Could you check a few things on this model? Use its own coordinates, in mm. Face numbers are marked on the shaded views. Give positions to 0.01 mm unless a question says otherwise; leave off trailing zeros. Loops run counter-clockwise (first coordinate to the right, second up) from the corner with the lowest first, then second, coordinate; pieces in that order, holes last. Notation, with made-up numbers: (60.5, 16.25) - (90.5, 16.25) arc R32 ccw to (90.5, 54.25) - close; hole circle Ø1 at (36, -3). An arc over 180 degrees is marked (long way). Write each question's results on one line, items separated by ' | '. Start each with the question number.
1) I want a section at D-D, the plane z = -5. Write out the boundary of the cut face in (x, y).
2) I want a section at B-B, the plane x = 0. Write out the boundary of the cut face in (y, z), and give its area (3 significant figures).
3) If we mould it in two halves opening along Y, with no side actions, what happens to the marked faces 1, 2 and 3? For each: +Y half, -Y half, draft (parallel to the pull), parting line (faces both ways), or undercut.
4) I'm going to push flat-ended pins straight in: pin 1 (6 mm diameter, centred on y = -17, z = 4, fed in from +X); pin 2 (2 mm diameter, centred on x = 1.5, y = -16, fed in from +Z); pin 3 (6 mm diameter, centred on x = -3.5, z = 4.5, fed in from -Y). Where does each tip first touch, or does it pass through?
5) If I drill on probe 1 along Y at (x, z) = (2.75, 2.25); probe 2 along Y at (x, z) = (5, -2.75); probe 3 along X at (y, z) = (-18.5, 6.5), over which ranges is the centre line in solid material (lowest first)? Write a range as [from, to].
6) I want a section at C-C, the plane y = -2. Write out the boundary of the cut face in (x, z), and give its area (3 significant figures).
7) I want a section at A-A, the plane z = 2.25. Write out the boundary of the cut face in (x, y).
from build123d import *

# Parameters (mm, degrees)
MOAR_SPRINGS_COUNT = 4
SKETCH13_R         = 1.27


with BuildPart() as part:
    # Sketch1 → button body (revolve)
    with BuildSketch(Plane.XY, mode=Mode.PRIVATE) as button_body_sk:
        Polygon((0, 0), (6.223, 0), (6.223, -5.08), (3.048, -5.08), (3.048, -10.16), (3.81, -10.16), (3.81, -12.7), (0, -12.7), align=None)
    revolve(button_body_sk.sketch.rotate(Axis((0, -12.7, 0), (0, 1, 0)), 90), axis=Axis((0, -12.7, 0), (0, 1, 0)))


with BuildPart() as moar_springs_1:
    # moar springs: pattern copy
    add(part.part.rotate(Axis((0, 0, 0), (0, -1, 0)), 1 * 360 / MOAR_SPRINGS_COUNT))


with BuildPart() as moar_springs_2:
    # moar springs: pattern copy
    add(part.part.rotate(Axis((0, 0, 0), (0, -1, 0)), 2 * 360 / MOAR_SPRINGS_COUNT))


with BuildPart() as moar_springs_3:
    # moar springs: pattern copy
    add(part.part.rotate(Axis((0, 0, 0), (0, -1, 0)), 3 * 360 / MOAR_SPRINGS_COUNT))


with BuildPart() as part_1:
    add(part.part)

    add(moar_springs_1.part)  # hook for baton merges moar springs_1

    add(moar_springs_2.part)  # hook for baton merges moar springs_2

    add(moar_springs_3.part)  # hook for baton merges moar springs_3
    # hook for baton: sweep along a path in Sketch12
    with BuildLine(Plane(origin=(0, 0, 0), x_dir=(0, 0, -1), z_dir=(1, 0, 0))) as hook_for_baton_path:
        Line((0, -12.7), (0, -16.51))
        ThreePointArc((0, -16.51), (-0.371974388, -17.408025612), (-1.27, -17.78))
        Line((-1.27, -17.78), (-5.08, -17.78))
        ThreePointArc((-5.08, -17.78), (-5.978025612, -17.408025612), (-6.35, -16.51))
        Line((-6.35, -16.51), (-6.35, -15.24))
    # Sketch13 → hook for baton (sweep)
    with BuildSketch(Plane(origin=(0, -12.7, 0), x_dir=(-1, 0, 0), z_dir=(0, -1, 0))):
        with Locations((0, 1.27)):
            Circle(SKETCH13_R)
    sweep(path=hook_for_baton_path.line)


solid = part_1.part
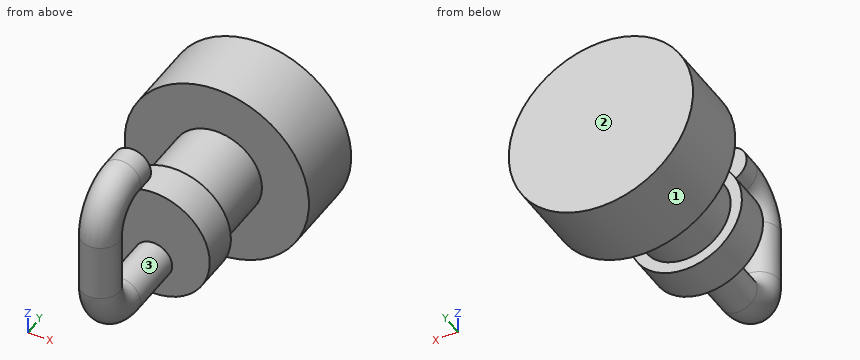
Answers:
1) outline: (-3.7, -5.08) - (3.7, -5.08) - (3.7, 0) - (-3.7, 0) - close
2) outline: (-20.32, 1.27) arc R3.81 ccw to (-16.51, -2.54) - (-12.7, -2.54) - (-12.7, -3.81) - (-10.16, -3.81) - (-10.16, -3.05) - (-5.08, -3.05) - (-5.08, -6.22) - (0, -6.22) - (0, 6.22) - (-5.08, 6.22) - (-5.08, 3.05) - (-10.16, 3.05) - (-10.16, 3.81) - (-12.7, 3.81) - (-12.7, 0) - (-16.51, 0) arc R1.27 cw to (-17.78, 1.27) - (-17.78, 5.08) arc R1.27 cw to (-16.51, 6.35) - (-15.24, 6.35) - (-15.24, 8.89) - (-16.51, 8.89) arc R3.81 ccw to (-20.32, 5.08) - close | area: 156 mm2
3) face 1: draft | face 2: +Y half | face 3: undercut
4) pin 1: stops at x = 1.27 | pin 2: stops at z = 8.79 | pin 3: stops at y = -20.22
5) probe 1: y = [-12.7, -10.16], [-5.08, 0] | probe 2: y = [-5.08, 0] | probe 3: x = [-1.27, 1.27]
6) outline: circle Ø12.45 at (0, 0) | area: 122 mm2
7) outline: (-5.8, -5.08) - (-2.06, -5.08) - (-2.06, -10.16) - (-3.07, -10.16) - (-3.07, -12.7) - (3.07, -12.7) - (3.07, -10.16) - (2.06, -10.16) - (2.06, -5.08) - (5.8, -5.08) - (5.8, 0) - (-5.8, 0) - close; circle Ø2.54 at (0, -19.05)
